```python
from build123d import *

# Parameters (mm, degrees)
EXTRUDE_1_DEPTH     = 7.5
CUT_EXTRUDE_1_DEPTH = 84.553874835
SHELL_1_T           = -1.5
CUT_EXTRUDE_START   = -2
CUT_EXTRUDE_2_DEPTH = 2
SKETCH_4_R          = 2.75
EXTRUDE_2_DEPTH     = 1.5
SKETCH_5_R          = 2
EXTRUDE_3_DEPTH     = 4.5
SKETCH_6_R          = 1.75
CUT_EXTRUDE_3_DEPTH = 2
SKETCH_9_R          = 1
CUT_EXTRUDE_4_DEPTH = 84.553874835
CUT_EXTRUDE_5_DEPTH = 84.553874835
SKETCH_12_W         = 1.5
SKETCH_12_H         = 12
CUT_EXTRUDE_6_DEPTH = 4.5


with BuildPart() as part:
    # 草图1 → 凸台-拉伸1 (new body)
    with BuildSketch(Plane.XY):
        with BuildLine():
            Line((-45, 70), (0, 70))
            Line((0, 70), (0, 8))
            ThreePointArc((0, 8), (-2.343145751, 2.343145751), (-8, 0))
            Line((-8, 0), (-37, 0))
            ThreePointArc((-37, 0), (-42.656854249, 2.343145751), (-45, 8))
            Line((-45, 8), (-45, 70))
        make_face()
    extrude(amount=EXTRUDE_1_DEPTH)

    # 草图2 → 切除-拉伸1 (cut, through all)
    with BuildSketch(Plane(origin=(0, 0, 0), x_dir=(0, 0, -1), z_dir=(1, 0, 0))):
        Polygon((0, 0), (0, 7.2), (-4, 0), align=None)
        Polygon((0, 70), (-1, 70), (0, 48), align=None)
    extrude(amount=-CUT_EXTRUDE_1_DEPTH, mode=Mode.SUBTRACT)

    # 抽壳1
    shell_1_openings = [part.faces().sort_by_distance(p)[0] for p in [
        (-22.5, 35.292176643, 7.5),
    ]]
    offset(amount=SHELL_1_T, openings=shell_1_openings, kind=Kind.INTERSECTION)

    # 草图3 → 切除-拉伸2 (cut)
    with BuildSketch(Plane.XY.offset(7.5).offset(CUT_EXTRUDE_START)):
        with BuildLine():
            Line((-44.25, 69.25), (-0.75, 69.25))
            Line((-0.75, 69.25), (-0.75, 8))
            ThreePointArc((-0.75, 8), (-2.873475836, 2.873475836), (-8, 0.75))
            Line((-8, 0.75), (-37, 0.75))
            ThreePointArc((-37, 0.75), (-42.126524164, 2.873475836), (-44.25, 8))
            Line((-44.25, 8), (-44.25, 69.25))
        make_face()
        with BuildLine():
            Line((-43.5, 68.5), (-1.5, 68.5))
            Line((-1.5, 68.5), (-1.5, 8))
            ThreePointArc((-1.5, 8), (-3.403805922, 3.403805922), (-8, 1.5))
            Line((-8, 1.5), (-37, 1.5))
            ThreePointArc((-37, 1.5), (-41.596194078, 3.403805922), (-43.5, 8))
            Line((-43.5, 8), (-43.5, 68.5))
        make_face(mode=Mode.SUBTRACT)
    extrude(amount=CUT_EXTRUDE_2_DEPTH, mode=Mode.SUBTRACT)

    # 草图4 → 凸台-拉伸2 (add)
    with BuildSketch(Plane.XY.offset(1.5)):
        with Locations(Location((-40.5, 65.5, 0), (0, 0, 270))):
            Circle(SKETCH_4_R)
        with Locations((-40.5, 5)):
            Circle(SKETCH_4_R)
        with Locations((-4.5, 5)):
            Circle(SKETCH_4_R)
        with Locations(Location((-4.5, 65.5, 0), (0, 0, 180))):
            Circle(SKETCH_4_R)
    extrude(amount=EXTRUDE_2_DEPTH)

    # 草图5 → 凸台-拉伸3 (add)
    with BuildSketch(Plane.XY.offset(3)):
        with Locations((-40.5, 65.5)):
            Circle(SKETCH_5_R)
        with Locations((-4.5, 65.5)):
            Circle(SKETCH_5_R)
        with Locations(Location((-40.5, 5, 0), (0, 0, 183.190472592))):
            Circle(SKETCH_5_R)
        with Locations(Location((-4.5, 5, 0), (0, 0, 183.190472592))):
            Circle(SKETCH_5_R)
    extrude(amount=EXTRUDE_3_DEPTH)

    # 草图6 → 切除-拉伸3 (cut)
    with BuildSketch(Plane(origin=(0, 0, 0), x_dir=(-1, 0, 0), z_dir=(0, 0, -1))):
        with Locations((4.5, 65.5)):
            Circle(SKETCH_6_R)
        with Locations((40.5, 65.5)):
            Circle(SKETCH_6_R)
        with Locations((40.5, 5)):
            Circle(SKETCH_6_R)
        with Locations((4.5, 5)):
            Circle(SKETCH_6_R)
    extrude(amount=-CUT_EXTRUDE_3_DEPTH, mode=Mode.SUBTRACT)

    # 草图9 → 切除-拉伸4 (cut, through all)
    with BuildSketch(Plane.XY):
        with Locations(Location((-40.5, 65.5, 0), (0, 0, 180))):
            Circle(SKETCH_9_R)
        with Locations(Location((-4.5, 65.5, 0), (0, 0, 180))):
            Circle(SKETCH_9_R)
        with Locations(Location((-4.5, 5, 0), (0, 0, 180))):
            Circle(SKETCH_9_R)
        with Locations(Location((-40.5, 5, 0), (0, 0, 180))):
            Circle(SKETCH_9_R)
    extrude(amount=CUT_EXTRUDE_4_DEPTH, mode=Mode.SUBTRACT)

    # 草图11 → 切除-拉伸5 (cut, through all)
    with BuildSketch(Plane(origin=(0, 0, 0), x_dir=(0, 0, -1), z_dir=(1, 0, 0))):
        Polygon((0, 0), (0, 7.2), (-4, 0), align=None)
        Polygon((0, 70), (-1, 70), (0, 48), align=None)
    extrude(amount=-CUT_EXTRUDE_5_DEPTH, mode=Mode.SUBTRACT)

    # 草图12 → 切除-拉伸6 (cut)
    with BuildSketch(Plane.XY.offset(7.5)):
        with Locations((-0.75, 56)):
            Rectangle(SKETCH_12_W, SKETCH_12_H)
    extrude(amount=-CUT_EXTRUDE_6_DEPTH, mode=Mode.SUBTRACT)


solid = part.part
```
The listing builds one solid part. Answer for the finished solid, in the listing's coordinates (mm). A direction names the side the tool comes from. Coordinates: 2 decimals unless noted, no trailing zeros. Loops run counter-clockwise (first coordinate to the right, second up) from the corner with the lowest first, then second, coordinate; pieces in that order, holes last. Notation, with made-up numbers: M -5.75,-33.5 L 35.25,-33.5 A24 cw 35.25,-16.5 Z; hole C 22.25,48.5 d6. An arc over 180 degrees is marked long. Answer as a JSON object with one key per item and string values. Group by question number.
Item 1: Section C-C (y = 51.5) is taken. Write down the section's boundary in (x, z), and give its area (3 significant figures).
Item 2: Each of these flat-tipped pins is pushed along its axis until it touches: P1, Ø1.8, axis at x = -41, y = 65, coming from the -Z side; P2, Ø4, axis at x = -26.5, y = 62, coming from the +Z side; P3, Ø2, axis at x = -39.5, y = 43.5, coming from the +Z side; P4, Ø1.2, axis at x = -40.5, y = 65.5, coming from the +Z side. Where does it stop, or does it pass through?
Item 3: Section A-A (z = 6.5) is taken. Give the number of separate pieces and of enclosed holes in the cut face, and give its area (3 significant figures).
Item 4: Section B-B (x = -31) is taken. Write down the section's boundary in (y, z).
Item 5: Consider L1, parallel to Y at x = -40.5, z = 1.15; L2, parallel to X at y = 65.5, z = 1.25; L3, parallel to Y at x = -33.5, z = 5.75. Determine where each line is inside the solid, lowest interval first.
Item 6: Which of the six approach directions +Z, -Z, +X, -X, +Y, -Y give full straight-line access (tool end or side, diameter ignored) to faces 3 (the face through (-1, 56, 3)), 4 (the face through (-23, 68.5, 4)), 5 (the face through (-22, 0, 6)), 6 (the face through (-5.3, 5.9, 2))?
Item 7: Determine the mould class of faces 1 (the face through (-22.185, 59.154, 0.507)), 2 (the face through (-4.142, 62.773, 2.662)) for opening direction X: +X half, -X half, draft (parallel to the pull), parting line (faces both ways), or undercut.
Solved:
{
 "1": {"outline": "M -45,0.16 L 0,0.16 L 0,3 L -1.5,3 L -1.5,1.66 L -43.5,1.66 L -43.5,5.5 L -44.25,5.5 L -44.25,7.5 L -45,7.5 Z", "area": "76.8 mm2"},
 "2": {"P1": "stops at z = 2", "P2": "stops at z = 2.23", "P3": "stops at z = 1.5", "P4": "passes through"},
 "3": {"separate pieces": "5", "enclosed holes": "4", "area": "194 mm2"},
 "4": {"outline": "M 0,4 L 7.2,0 L 48,0 L 70,1 L 70,7.5 L 69.25,7.5 L 69.25,5.5 L 68.5,5.5 L 68.5,2.43 L 47.97,1.5 L 7.59,1.5 L 1.5,4.88 L 1.5,5.5 L 0.75,5.5 L 0.75,7.5 L 0,7.5 Z"},
 "5": {"L1": "y = 6.75 to 63.75, 67.25 to 70", "L2": "x = -45 to -42.25, -38.75 to -6.25, -2.75 to 0", "L3": "y = 0 to 0.75, 69.25 to 70"},
 "6": {"face 3": "+Z, +X", "face 4": "+Z", "face 5": "+Z, -Z, +X, -X, -Y", "face 6": "-Z"},
 "7": {"face 1": "draft", "face 2": "undercut"}
}
